from build123d import *


with BuildPart() as part:
    # ProfileS → Profile (revolve)
    with BuildSketch(Plane.XY):
        with BuildLine():
            Line((0, 0), (90.093578278, 0))
            ThreePointArc((90.093578278, 0), (94.284750443, 0.64207816), (98.091485449, 2.509417731))
            Line((98.091485449, 2.509417731), (124.785639542, 21.089622062))
            ThreePointArc((124.785639542, 21.089622062), (124.977068637, 21.64968472), (124.5, 22))
            Line((124.5, 22), (122.344952056, 22))
            ThreePointArc((122.344952056, 22), (121.746213175, 21.908274549), (121.202393889, 21.641511753))
            Line((121.202393889, 21.641511753), (96.66328774, 4.561307422))
            ThreePointArc((96.66328774, 4.561307422), (93.536326842, 3.027421346), (90.093578278, 2.5))
            Line((90.093578278, 2.5), (0, 2.5))
            Line((0, 2.5), (0, 0))
        make_face()
    revolve(axis=Axis((0, 0, 0), (0, 1, 0)))


solid = part.part
For this review, take the finished solid that the model builds, in its own axes (mm). Round coordinates to 2 decimals unless told otherwise and drop trailing zeros. Order: outer loops, then holes, each group sorted by start corner. A loop starts at its lowest first (then second) coordinate and runs counter-clockwise, first axis right, second up. Notation, with made-up numbers: M -15,84.25 L -2,84.25 A34 ccw -2,115.25 Z; hole C 20,-38.5 d6. An arc over 180 degrees is marked long. Use a Markdown table: item, result. Add a question column.
Item 1: Mouldability with a two-part tool opening along Z and no side actions: class faces 1 (the flat face through (1, 0, -1)), 2 (the conical face through (92.2, 3.7, 38.2)), 3 (the flat face through (-1, 2.5, -1)) as released by +Z, released by -Z, zero draft, split by the parting line, or undercut.
Item 2: Add section A-A, the plane x = 0. Give the boundary of the cut face in (y, z).
Item 3: Insertion check: pin 1 (6 mm diameter, centred on x = 79, y = 7, fed in from -Z); pin 2 (1 mm diameter, centred on y = 9.5, z = -28.5, fed in from -X); pin 3 (1.5 mm diameter, centred on x = 11, z = -90, fed in from +Y). Each pin has a flat end and moves straight along its axis. Give the tip position at first contact, or say it passes through.
Item 4: Add section C-C, the plane y = 14.75. Give the boundary of the cut face in (x, z).
Item 5: To check wall thickness, follow line 1 along Y through (x, z) = (-50.5, 14.5); line 2 along Z through (x, y) = (58, 6); line 3 along X through (y, z) = (21.25, -36). State the ranges of each line that lie inside material, in increasing order.
Item 6: Add section B-B, the plane z = 0. Give the boundary of the cut face in (x, y).
Geometry results:
| question | item | result |
|---|---|---|
| 1 | face 1 | zero draft |
| 1 | face 2 | split by the parting line |
| 1 | face 3 | undercut |
| 2 | outline | M 0,-90.09 A14 ccw 2.51,-98.09 L 21.09,-124.79 A0.5 ccw 22,-124.5 L 22,-122.34 A2 ccw 21.64,-121.2 L 4.56,-96.66 A11.5 cw 2.5,-90.09 L 2.5,90.09 A11.5 cw 4.56,96.66 L 21.64,121.2 A2 ccw 22,122.34 L 22,124.5 A0.5 ccw 21.09,124.79 L 2.51,98.09 A14 ccw 0,90.09 Z |
| 3 | pin 1 | stops at z = -75.63 |
| 3 | pin 2 | stops at x = -105.07 |
| 3 | pin 3 | stops at y = 2.58 |
| 4 | outline | C 0,0 d231.36; hole C 0,0 d222.6 |
| 5 | line 1 | y = 0 to 2.5 |
| 5 | line 2 | z = -85.25 to -79.9, 79.9 to 85.25 |
| 5 | line 3 | x = -119.63 to -115.14, 115.14 to 119.63 |
| 6 | outline | M -124.79,21.09 L -98.09,2.51 A14 ccw -90.09,0 L 90.09,0 A14 ccw 98.09,2.51 L 124.79,21.09 A0.5 ccw 124.5,22 L 122.34,22 A2 ccw 121.2,21.64 L 96.66,4.56 A11.5 cw 90.09,2.5 L -90.09,2.5 A11.5 cw -96.66,4.56 L -121.2,21.64 A2 ccw -122.34,22 L -124.5,22 A0.5 ccw Z |
